For this review, use the dimensioned drawing (mm, ordinates from the lowest corner) and the shaded views. A direction names the side the tool comes from. Coordinates: 2 decimals unless noted, no trailing zeros. Order: outer loops, then holes, each group sorted by start corner. A loop starts at its lowest first (then second) coordinate and runs counter-clockwise, first axis right, second up. Notation, with made-up numbers: M 17,-10.75 L 36,-10.75 A28 ccw 36,8.25 Z; hole C 68.5,39 d10. An arc over 180 degrees is marked long. One line per item, written item: value.
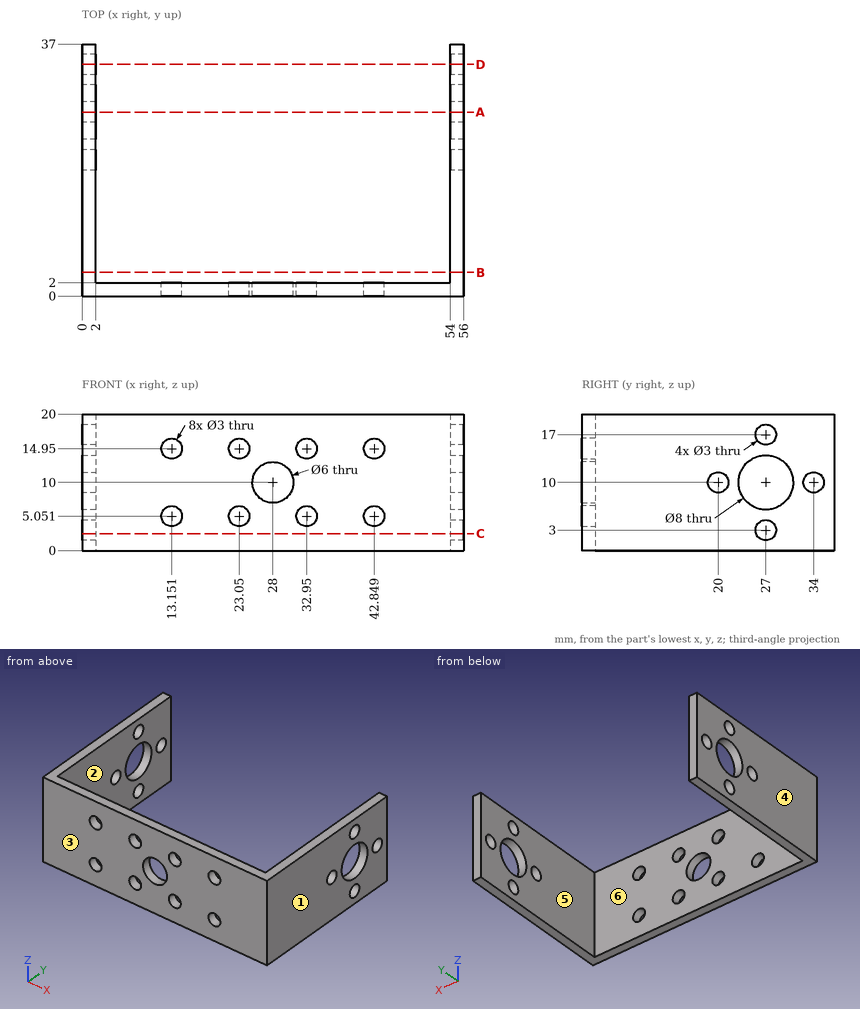
(1) Mouldability with a two-part tool opening along X and no side actions: class the marked faces 3, 4, 5 and 6 as +X half, -X half, draft (parallel to the pull), parting line (faces both ways), or undercut.
Geometry results:
face 3: draft
face 4: -X half
face 5: undercut
face 6: undercut
(2) We need section B-B, the plane y = 3.5. State the section outline as (x, z) points.
Geometry results:
outline: M 0,0 L 2,0 L 2,20 L 0,20 Z; M 54,0 L 56,0 L 56,20 L 54,20 Z
(3) Insertion check: pin 1 Ø3 at (x, z) = (24, 13.5) entering from +Y. The pin has a flat end and moves straight along its axis. Give the tip position at first contact, or say it passes through.
Geometry results:
pin 1: stops at y = 2
(4) We need section C-C, the plane z = 2.5. State the section outline as (x, y) points (1 decimal).
Geometry results:
outline: M 0,0 L 56,0 L 56,25.6 L 54,25.6 L 54,2 L 2,2 L 2,25.6 L 0,25.6 Z; M 0,28.4 L 2,28.4 L 2,37 L 0,37 Z; M 54,28.4 L 56,28.4 L 56,37 L 54,37 Z
(5) For L1, parallel to X at y = 15, z = 1.5; L2, parallel to Y at x = 1, z = 10; L3, parallel to Y at x = 0.65, z = 17, list the stretches that pass through material, from the lowest coordinate up.
Geometry results:
L1: x = 0 to 2, 54 to 56
L2: y = 0 to 18.5, 21.5 to 23, 31 to 32.5, 35.5 to 37
L3: y = 0 to 25.5, 28.5 to 37
(6) We need section A-A, the plane y = 27. Count the separate pieces of the cut face and the enclosed holes in it.
Geometry results:
separate pieces: 8
enclosed holes: 0
(7) Tool access review of the marked faces 1 and 2: name each direction out of +Z, -Z, +X, -X, +Y, -Y from which nothing blocks a thin tool from reaching the whole face with its end or side.
Geometry results:
face 1: +Z, -Z, +X, +Y, -Y
face 2: +Z, -Z, +Y
(8) We need section D-D, the plane y = 34. State the section outline as (x, z) points.
Geometry results:
outline: M 0,0 L 2,0 L 2,8.5 L 0,8.5 Z; M 0,11.5 L 2,11.5 L 2,20 L 0,20 Z; M 54,0 L 56,0 L 56,8.5 L 54,8.5 Z; M 54,11.5 L 56,11.5 L 56,20 L 54,20 Z
